```python
from build123d import *

# Parameters (mm, degrees)
SKETCH1_W           = 49.2
SKETCH1_H           = 37.6
BOSS_EXTRUDE1_DEPTH = 2
SKETCH2_W           = 2
SKETCH2_H           = 37.6
BOSS_EXTRUDE2_DEPTH = 37.6
BOSS_EXTRUDE5_DEPTH = 37.6
CUT_EXTRUDE1_REACH  = 78.051
SKETCH4_R           = 1.55
FILLET2_R           = 5
CUT_EXTRUDE2_REACH  = 70.887
SKETCH5_R           = 1.65
CUT_EXTRUDE3_START  = -2
CUT_EXTRUDE3_DEPTH  = 2
CUT_EXTRUDE4_REACH  = 70.887


# Read off the part's stored shape, not the designer's step: Cut-Extrude3
with BuildPart() as part:
    # Sketch1 → Boss-Extrude1 (new body)
    with BuildSketch(Plane(origin=(0, 0, 0), x_dir=(1, 0, 0), z_dir=(0, 1, 0))):
        with Locations((-33.511891694, -8.706295402)):
            Rectangle(SKETCH1_W, SKETCH1_H)
    extrude(amount=BOSS_EXTRUDE1_DEPTH)



with BuildPart() as body_2:
    # Sketch2 → Boss-Extrude2 (new body)
    with BuildSketch(Plane(origin=(0, 2, 0), x_dir=(1, 0, 0), z_dir=(0, 1, 0))):
        with Locations((-59.111891694, -8.706295402)):
            Rectangle(SKETCH2_W, SKETCH2_H)
    extrude(amount=BOSS_EXTRUDE2_DEPTH)


with BuildPart() as part_1:
    add(part.part)

    add(body_2.part)  # Boss-Extrude5 merges body 2
    # Sketch3 → Boss-Extrude5 (add)
    with BuildSketch(Plane.XY.offset(27.506295402)):
        with BuildLine():
            Line((-60.111891694, 2), (-58.111891694, 2))
            Line((-58.111891694, 2), (-58.111891694, 0))
            ThreePointArc((-58.111891694, 0), (-59.526105257, 0.585786438), (-60.111891694, 2))
        make_face()
    extrude(amount=-BOSS_EXTRUDE5_DEPTH)

    # Sketch4 → Cut-Extrude1 (cut, up to next)
    with BuildSketch(Plane(origin=(0, 2, 0), x_dir=(1, 0, 0), z_dir=(0, 1, 0)), mode=Mode.PRIVATE) as cut_extrude1_sk1:
        with Locations(Location((-51.711891694, 6.893704598, 0), (0, 0, 270))):
            Circle(SKETCH4_R)
    cut_extrude1_tool1 = extrude(cut_extrude1_sk1.sketch, amount=-CUT_EXTRUDE1_REACH, mode=Mode.PRIVATE) & part_1.part
    # Sketch4 → Cut-Extrude1 (cut, up to next)
    with BuildSketch(Plane(origin=(0, 2, 0), x_dir=(1, 0, 0), z_dir=(0, 1, 0)), mode=Mode.PRIVATE) as cut_extrude1_sk2:
        with Locations(Location((-51.711891694, -24.306295402, 0), (0, 0, 270))):
            Circle(SKETCH4_R)
    cut_extrude1_tool2 = extrude(cut_extrude1_sk2.sketch, amount=-CUT_EXTRUDE1_REACH, mode=Mode.PRIVATE) & part_1.part
    # Sketch4 → Cut-Extrude1 (cut, up to next)
    with BuildSketch(Plane(origin=(0, 2, 0), x_dir=(1, 0, 0), z_dir=(0, 1, 0)), mode=Mode.PRIVATE) as cut_extrude1_sk3:
        with Locations(Location((-45.311891694, 6.893704598, 0), (0, 0, 270))):
            Circle(SKETCH4_R)
    cut_extrude1_tool3 = extrude(cut_extrude1_sk3.sketch, amount=-CUT_EXTRUDE1_REACH, mode=Mode.PRIVATE) & part_1.part
    # Sketch4 → Cut-Extrude1 (cut, up to next)
    with BuildSketch(Plane(origin=(0, 2, 0), x_dir=(1, 0, 0), z_dir=(0, 1, 0)), mode=Mode.PRIVATE) as cut_extrude1_sk4:
        with Locations(Location((-38.911891694, 6.893704598, 0), (0, 0, 270))):
            Circle(SKETCH4_R)
    cut_extrude1_tool4 = extrude(cut_extrude1_sk4.sketch, amount=-CUT_EXTRUDE1_REACH, mode=Mode.PRIVATE) & part_1.part
    # Sketch4 → Cut-Extrude1 (cut, up to next)
    with BuildSketch(Plane(origin=(0, 2, 0), x_dir=(1, 0, 0), z_dir=(0, 1, 0)), mode=Mode.PRIVATE) as cut_extrude1_sk5:
        with Locations(Location((-32.511891694, 6.893704598, 0), (0, 0, 270))):
            Circle(SKETCH4_R)
    cut_extrude1_tool5 = extrude(cut_extrude1_sk5.sketch, amount=-CUT_EXTRUDE1_REACH, mode=Mode.PRIVATE) & part_1.part
    # Sketch4 → Cut-Extrude1 (cut, up to next)
    with BuildSketch(Plane(origin=(0, 2, 0), x_dir=(1, 0, 0), z_dir=(0, 1, 0)), mode=Mode.PRIVATE) as cut_extrude1_sk6:
        with Locations(Location((-26.111891694, 6.893704598, 0), (0, 0, 270))):
            Circle(SKETCH4_R)
    cut_extrude1_tool6 = extrude(cut_extrude1_sk6.sketch, amount=-CUT_EXTRUDE1_REACH, mode=Mode.PRIVATE) & part_1.part
    # Sketch4 → Cut-Extrude1 (cut, up to next)
    with BuildSketch(Plane(origin=(0, 2, 0), x_dir=(1, 0, 0), z_dir=(0, 1, 0)), mode=Mode.PRIVATE) as cut_extrude1_sk7:
        with Locations(Location((-19.711891694, 6.893704598, 0), (0, 0, 270))):
            Circle(SKETCH4_R)
    cut_extrude1_tool7 = extrude(cut_extrude1_sk7.sketch, amount=-CUT_EXTRUDE1_REACH, mode=Mode.PRIVATE) & part_1.part
    # Sketch4 → Cut-Extrude1 (cut, up to next)
    with BuildSketch(Plane(origin=(0, 2, 0), x_dir=(1, 0, 0), z_dir=(0, 1, 0)), mode=Mode.PRIVATE) as cut_extrude1_sk8:
        with Locations(Location((-13.311891694, 6.893704598, 0), (0, 0, 270))):
            Circle(SKETCH4_R)
    cut_extrude1_tool8 = extrude(cut_extrude1_sk8.sketch, amount=-CUT_EXTRUDE1_REACH, mode=Mode.PRIVATE) & part_1.part
    # Sketch4 → Cut-Extrude1 (cut, up to next)
    with BuildSketch(Plane(origin=(0, 2, 0), x_dir=(1, 0, 0), z_dir=(0, 1, 0)), mode=Mode.PRIVATE) as cut_extrude1_sk9:
        with Locations(Location((-13.311891694, -24.306295402, 0), (0, 0, 270))):
            Circle(SKETCH4_R)
    cut_extrude1_tool9 = extrude(cut_extrude1_sk9.sketch, amount=-CUT_EXTRUDE1_REACH, mode=Mode.PRIVATE) & part_1.part
    # Sketch4 → Cut-Extrude1 (cut, up to next)
    with BuildSketch(Plane(origin=(0, 2, 0), x_dir=(1, 0, 0), z_dir=(0, 1, 0)), mode=Mode.PRIVATE) as cut_extrude1_sk10:
        with Locations(Location((-19.711891694, -24.306295402, 0), (0, 0, 270))):
            Circle(SKETCH4_R)
    cut_extrude1_tool10 = extrude(cut_extrude1_sk10.sketch, amount=-CUT_EXTRUDE1_REACH, mode=Mode.PRIVATE) & part_1.part
    # Sketch4 → Cut-Extrude1 (cut, up to next)
    with BuildSketch(Plane(origin=(0, 2, 0), x_dir=(1, 0, 0), z_dir=(0, 1, 0)), mode=Mode.PRIVATE) as cut_extrude1_sk11:
        with Locations(Location((-26.111891694, -24.306295402, 0), (0, 0, 270))):
            Circle(SKETCH4_R)
    cut_extrude1_tool11 = extrude(cut_extrude1_sk11.sketch, amount=-CUT_EXTRUDE1_REACH, mode=Mode.PRIVATE) & part_1.part
    # Sketch4 → Cut-Extrude1 (cut, up to next)
    with BuildSketch(Plane(origin=(0, 2, 0), x_dir=(1, 0, 0), z_dir=(0, 1, 0)), mode=Mode.PRIVATE) as cut_extrude1_sk12:
        with Locations(Location((-32.511891694, -24.306295402, 0), (0, 0, 270))):
            Circle(SKETCH4_R)
    cut_extrude1_tool12 = extrude(cut_extrude1_sk12.sketch, amount=-CUT_EXTRUDE1_REACH, mode=Mode.PRIVATE) & part_1.part
    # Sketch4 → Cut-Extrude1 (cut, up to next)
    with BuildSketch(Plane(origin=(0, 2, 0), x_dir=(1, 0, 0), z_dir=(0, 1, 0)), mode=Mode.PRIVATE) as cut_extrude1_sk13:
        with Locations(Location((-38.911891694, -24.306295402, 0), (0, 0, 270))):
            Circle(SKETCH4_R)
    cut_extrude1_tool13 = extrude(cut_extrude1_sk13.sketch, amount=-CUT_EXTRUDE1_REACH, mode=Mode.PRIVATE) & part_1.part
    # Sketch4 → Cut-Extrude1 (cut, up to next)
    with BuildSketch(Plane(origin=(0, 2, 0), x_dir=(1, 0, 0), z_dir=(0, 1, 0)), mode=Mode.PRIVATE) as cut_extrude1_sk14:
        with Locations(Location((-45.311891694, -24.306295402, 0), (0, 0, 270))):
            Circle(SKETCH4_R)
    cut_extrude1_tool14 = extrude(cut_extrude1_sk14.sketch, amount=-CUT_EXTRUDE1_REACH, mode=Mode.PRIVATE) & part_1.part
    add(cut_extrude1_tool1.solids().sort_by_distance((-51.711892, 2, -6.893705))[0], mode=Mode.SUBTRACT)
    add(cut_extrude1_tool2.solids().sort_by_distance((-51.711892, 2, 24.306295))[0], mode=Mode.SUBTRACT)
    add(cut_extrude1_tool3.solids().sort_by_distance((-45.311892, 2, -6.893705))[0], mode=Mode.SUBTRACT)
    add(cut_extrude1_tool4.solids().sort_by_distance((-38.911892, 2, -6.893705))[0], mode=Mode.SUBTRACT)
    add(cut_extrude1_tool5.solids().sort_by_distance((-32.511892, 2, -6.893705))[0], mode=Mode.SUBTRACT)
    add(cut_extrude1_tool6.solids().sort_by_distance((-26.111892, 2, -6.893705))[0], mode=Mode.SUBTRACT)
    add(cut_extrude1_tool7.solids().sort_by_distance((-19.711892, 2, -6.893705))[0], mode=Mode.SUBTRACT)
    add(cut_extrude1_tool8.solids().sort_by_distance((-13.311892, 2, -6.893705))[0], mode=Mode.SUBTRACT)
    add(cut_extrude1_tool9.solids().sort_by_distance((-13.311892, 2, 24.306295))[0], mode=Mode.SUBTRACT)
    add(cut_extrude1_tool10.solids().sort_by_distance((-19.711892, 2, 24.306295))[0], mode=Mode.SUBTRACT)
    add(cut_extrude1_tool11.solids().sort_by_distance((-26.111892, 2, 24.306295))[0], mode=Mode.SUBTRACT)
    add(cut_extrude1_tool12.solids().sort_by_distance((-32.511892, 2, 24.306295))[0], mode=Mode.SUBTRACT)
    add(cut_extrude1_tool13.solids().sort_by_distance((-38.911892, 2, 24.306295))[0], mode=Mode.SUBTRACT)
    add(cut_extrude1_tool14.solids().sort_by_distance((-45.311892, 2, 24.306295))[0], mode=Mode.SUBTRACT)

    # Fillet2
    fillet2_edges = [part_1.edges().sort_by_distance(p)[0] for p in [
        (-8.911891694, 1, 27.506295402),
        (-8.911891694, 1, -10.093704598),
    ]]
    fillet(fillet2_edges, radius=FILLET2_R)

    # Sketch5 → Cut-Extrude2 (cut, up to next)
    with BuildSketch(Plane(origin=(-58.111891694, 0, 0), x_dir=(0, 0, -1), z_dir=(1, 0, 0)), mode=Mode.PRIVATE) as cut_extrude2_sk1:
        with Locations((6.793704598, 20.8)):
            Circle(SKETCH5_R)
    cut_extrude2_tool1 = extrude(cut_extrude2_sk1.sketch, amount=-CUT_EXTRUDE2_REACH, mode=Mode.PRIVATE) & part_1.part
    # Sketch5 → Cut-Extrude2 (cut, up to next)
    with BuildSketch(Plane(origin=(-58.111891694, 0, 0), x_dir=(0, 0, -1), z_dir=(1, 0, 0)), mode=Mode.PRIVATE) as cut_extrude2_sk2:
        with Locations((-0.956295402, 7.376606241)):
            Circle(SKETCH5_R)
    cut_extrude2_tool2 = extrude(cut_extrude2_sk2.sketch, amount=-CUT_EXTRUDE2_REACH, mode=Mode.PRIVATE) & part_1.part
    # Sketch5 → Cut-Extrude2 (cut, up to next)
    with BuildSketch(Plane(origin=(-58.111891694, 0, 0), x_dir=(0, 0, -1), z_dir=(1, 0, 0)), mode=Mode.PRIVATE) as cut_extrude2_sk3:
        with Locations((-16.456295402, 7.376606241)):
            Circle(SKETCH5_R)
    cut_extrude2_tool3 = extrude(cut_extrude2_sk3.sketch, amount=-CUT_EXTRUDE2_REACH, mode=Mode.PRIVATE) & part_1.part
    # Sketch5 → Cut-Extrude2 (cut, up to next)
    with BuildSketch(Plane(origin=(-58.111891694, 0, 0), x_dir=(0, 0, -1), z_dir=(1, 0, 0)), mode=Mode.PRIVATE) as cut_extrude2_sk4:
        with Locations((-24.206295402, 20.8)):
            Circle(SKETCH5_R)
    cut_extrude2_tool4 = extrude(cut_extrude2_sk4.sketch, amount=-CUT_EXTRUDE2_REACH, mode=Mode.PRIVATE) & part_1.part
    # Sketch5 → Cut-Extrude2 (cut, up to next)
    with BuildSketch(Plane(origin=(-58.111891694, 0, 0), x_dir=(0, 0, -1), z_dir=(1, 0, 0)), mode=Mode.PRIVATE) as cut_extrude2_sk5:
        with Locations((-16.456295402, 34.223393759)):
            Circle(SKETCH5_R)
    cut_extrude2_tool5 = extrude(cut_extrude2_sk5.sketch, amount=-CUT_EXTRUDE2_REACH, mode=Mode.PRIVATE) & part_1.part
    # Sketch5 → Cut-Extrude2 (cut, up to next)
    with BuildSketch(Plane(origin=(-58.111891694, 0, 0), x_dir=(0, 0, -1), z_dir=(1, 0, 0)), mode=Mode.PRIVATE) as cut_extrude2_sk6:
        with Locations((-0.956295402, 34.223393759)):
            Circle(SKETCH5_R)
    cut_extrude2_tool6 = extrude(cut_extrude2_sk6.sketch, amount=-CUT_EXTRUDE2_REACH, mode=Mode.PRIVATE) & part_1.part
    add(cut_extrude2_tool1.solids().sort_by_distance((-58.111892, 20.8, -6.793705))[0], mode=Mode.SUBTRACT)
    add(cut_extrude2_tool2.solids().sort_by_distance((-58.111892, 7.376606, 0.956295))[0], mode=Mode.SUBTRACT)
    add(cut_extrude2_tool3.solids().sort_by_distance((-58.111892, 7.376606, 16.456295))[0], mode=Mode.SUBTRACT)
    add(cut_extrude2_tool4.solids().sort_by_distance((-58.111892, 20.8, 24.206295))[0], mode=Mode.SUBTRACT)
    add(cut_extrude2_tool5.solids().sort_by_distance((-58.111892, 34.223394, 16.456295))[0], mode=Mode.SUBTRACT)
    add(cut_extrude2_tool6.solids().sort_by_distance((-58.111892, 34.223394, 0.956295))[0], mode=Mode.SUBTRACT)

    # Cut-Extrude3 outline → Cut-Extrude3 (cut)
    with BuildSketch(Plane(origin=(-58.111891694, 0, 0), x_dir=(0, 0, -1), z_dir=(1, 0, 0)).offset(CUT_EXTRUDE3_START)):
        with BuildLine():
            Line((-27.506295402, 39.6), (-27.506295402, 20.8))
            ThreePointArc((-27.506295402, 20.8), (-21.999902888, 34.093607486), (-8.706295402, 39.6))
            Line((-8.706295402, 39.6), (-27.506295402, 39.6))
        make_face()
        with BuildLine():
            Line((10.093704598, 39.6), (-8.706295402, 39.6))
            ThreePointArc((-8.706295402, 39.6), (4.587312084, 34.093607486), (10.093704598, 20.8))
            Line((10.093704598, 20.8), (10.093704598, 39.6))
        make_face()
    extrude(amount=CUT_EXTRUDE3_DEPTH, mode=Mode.SUBTRACT)

    # Sketch8 → Cut-Extrude4 (cut, up to next)
    with BuildSketch(Plane(origin=(-58.111891694, 0, 0), x_dir=(0, 0, -1), z_dir=(1, 0, 0)), mode=Mode.PRIVATE) as cut_extrude4_sk1:
        with BuildLine():
            Line((-15.294989136, 13.7999966), (-15.294989136, 27.7999966))
            ThreePointArc((-15.294989136, 27.7999966), (-8.694989136, 34.3999966), (-2.094989136, 27.7999966))
            Line((-2.094989136, 27.7999966), (-2.094989136, 13.7999966))
            ThreePointArc((-2.094989136, 13.7999966), (-8.694989136, 7.1999966), (-15.294989136, 13.7999966))
        make_face()
    cut_extrude4_tool1 = extrude(cut_extrude4_sk1.sketch, amount=-CUT_EXTRUDE4_REACH, mode=Mode.PRIVATE) & part_1.part
    add(cut_extrude4_tool1.solids().sort_by_distance((-58.111892, 20.799997, 8.694989))[0], mode=Mode.SUBTRACT)


solid = part_1.part
```
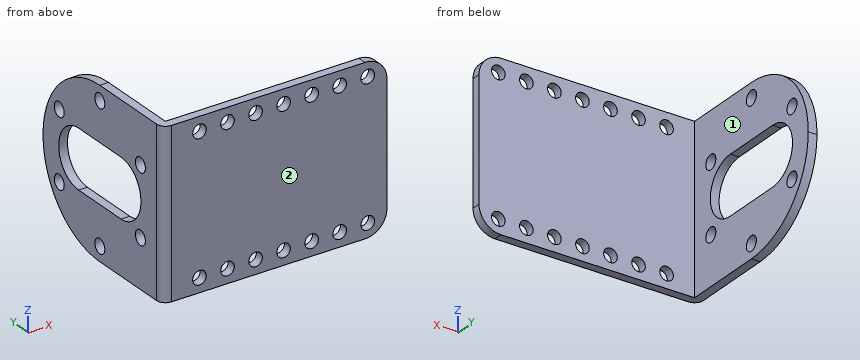
Part model, mm, in its own coordinate system. Face numbers are marked on the shaded views. A direction names the side the tool comes from. Give positions to 0.01 mm unless a question says otherwise; leave off trailing zeros. Order: outer loops, then holes, each group sorted by start corner. A loop starts at its lowest first (then second) coordinate and runs counter-clockwise, first axis right, second up. Notation, with made-up numbers: M 27.25,21 L 81.25,21 A36 cw 81.25,57 Z; hole C -21.75,-12.5 d8. An arc over 180 degrees is marked long. Use a Markdown table: item, result. Add a question column.
(1) Drop flat-ended pins along their axis: P1, Ø1.5, axis at y = 35, z = 3, coming from the +X side; P2, Ø19, axis at x = -41.5, z = 5, coming from the +Y side; P3, Ø1, axis at x = -58.5, y = 23.5, coming from the -Z side. Give the stop position or say it passes through.
(2) Saw through at B-B, the plane z = 6. Give the cut face in (x, y), and give its area (3 significant figures).
(3) Saw through at A-A, the plane y = 18. Give the cut face in (x, z).
(4) Saw through at D-D, the plane y = 24. Give the cut face in (x, z), and give its area (3 significant figures).
(5) Saw through at C-C, the plane z = 0. Give the cut face in (x, y).
(6) Probe line 1 along Y through (x, z) = (-53.5, -3.5); line 2 along X through (y, z) = (31, -2). List the from-to ranges inside material, lowest first. Write a range as [from, to].
(7) 3-axis set-ups, long thin cutter, end or side, ignore diameter. For the marked faces 1 and 2: which of +Z, -Z, +X, -X, +Y, -Y reach the whole face in a straight line?
Answer key:
| question | item | result |
|---|---|---|
| 1 | P1 | x = -58.11 |
| 1 | P2 | y = 2 |
| 1 | P3 | z = -9.96 |
| 2 | outline | M -60.11,2 A2 ccw -58.11,0 L -8.91,0 L -8.91,2 L -58.11,2 L -58.11,7.78 L -60.11,7.78 Z; M -60.11,33.82 L -58.11,33.82 L -58.11,39.4 L -60.11,39.4 Z |
| 2 | area | 124 mm^2 |
| 3 | outline | M -60.11,-10.09 L -58.11,-10.09 L -58.11,2.09 L -60.11,2.09 Z; M -60.11,15.29 L -58.11,15.29 L -58.11,27.51 L -60.11,27.51 Z |
| 4 | outline | M -60.11,-9.82 L -58.11,-9.82 L -58.11,2.09 L -60.11,2.09 Z; M -60.11,15.29 L -58.11,15.29 L -58.11,27.23 L -60.11,27.23 Z |
| 4 | area | 47.7 mm^2 |
| 5 | outline | M -60.11,2 A2 ccw -58.11,0 L -8.91,0 L -8.91,2 L -58.11,2 L -58.11,6.03 L -60.11,6.03 Z; M -60.11,8.72 L -58.11,8.72 L -58.11,32.88 L -60.11,32.88 Z; M -60.11,35.57 L -58.11,35.57 L -58.11,37.46 L -60.11,37.46 Z |
| 6 | line 1 | [0, 2] |
| 6 | line 2 | [-60.11, -58.11] |
| 7 | face 1 | +Z, -Z, +X, +Y |
| 7 | face 2 | +Z, -Z, +X, -X, -Y |
